The listing builds one solid part. Answer for the finished solid, in the listing's coordinates (mm). A direction names the side the tool comes from. Coordinates: 2 decimals unless noted, no trailing zeros. Write each loop counter-clockwise with the first axis right and the second up, starting at its lowest first coordinate (ties: lowest second). Pieces come first, ordered by that corner, then holes. Notation, with made-up numbers: M 18,79.5 L 53,79.5 A31 cw 53,105.5 Z; hole C 86,7 d2. An arc over 180 degrees is marked long. Answer as a JSON object with one key per item and string values. Group by question number.
from build123d import *

# Parameters (mm, degrees)
SKETCH2_R               = 101.6
BOSS_EXTRUDE1_DEPTH     = 76.2
SKETCH3_R               = 19.05
BOSS_EXTRUDE2_DEPTH     = 330.2
SKETCH12_R              = 20.32
BOSS_EXTRUDE5_DEPTH     = 7.62
BOSS_EXTRUDE6_OUTLINE_R = 19.05
BOSS_EXTRUDE6_DEPTH     = 35.56
SKETCH14_R              = 20.32
BOSS_EXTRUDE7_DEPTH     = 7.62
BOSS_EXTRUDE8_OUTLINE_R = 19.05
BOSS_EXTRUDE8_DEPTH     = 254
SKETCH16_R              = 101.6
BOSS_EXTRUDE9_DEPTH     = 76.2


# Read off the part's stored shape, not the designer's step: Boss-Extrude6, Boss-Extrude8
with BuildPart() as part:
    # Sketch2 → Boss-Extrude1 (new body)
    with BuildSketch(Plane.XY):
        with Locations(Location((0, 0, 0), (0, 0, 180))):
            Circle(SKETCH2_R)
    extrude(amount=BOSS_EXTRUDE1_DEPTH)

    # Sketch3 → Boss-Extrude2 (add)
    with BuildSketch(Plane.XY):
        Circle(SKETCH3_R)
    extrude(amount=BOSS_EXTRUDE2_DEPTH)

    # Sketch12 → Boss-Extrude5 (add)
    with BuildSketch(Plane.XY.offset(330.2)):
        with Locations(Location((0, 0, 0), (0, 0, 180))):
            Circle(SKETCH12_R)
    extrude(amount=BOSS_EXTRUDE5_DEPTH)

    # Boss-Extrude6 outline → Boss-Extrude6 (add)
    with BuildSketch(Plane.XY.offset(337.82)):
        Circle(BOSS_EXTRUDE6_OUTLINE_R)
    extrude(amount=BOSS_EXTRUDE6_DEPTH)

    # Sketch14 → Boss-Extrude7 (add)
    with BuildSketch(Plane.XY.offset(373.38)):
        with Locations(Location((0, 0, 0), (0, 0, 180))):
            Circle(SKETCH14_R)
    extrude(amount=BOSS_EXTRUDE7_DEPTH)

    # Boss-Extrude8 outline → Boss-Extrude8 (add)
    with BuildSketch(Plane.XY.offset(381)):
        Circle(BOSS_EXTRUDE8_OUTLINE_R)
    extrude(amount=BOSS_EXTRUDE8_DEPTH)

    # Sketch16 → Boss-Extrude9 (add)
    with BuildSketch(Plane.XY.offset(635)):
        with Locations(Location((0, 0, 0), (0, 0, 180))):
            Circle(SKETCH16_R)
    extrude(amount=BOSS_EXTRUDE9_DEPTH)


solid = part.part
Item 1: Consider L1, parallel to Z at x = 7, y = -47; L2, parallel to X at y = 1, z = 520; L3, parallel to Y at x = 2.5, z = 63. Determine where each line is inside the solid, lowest interval first. Write a range as from..to.
Item 2: A cutting plane is placed at B-B, the plane x = 0. Write down the section's boundary in (y, z), and give its area (3 significant figures).
Item 3: For a pull along Z with two mould halves and no side action, classify faces 3 (the face through (2.645, -20.147, 377.137)), 4 (the face through (-1, 1, 0)), 5 (the face through (-46.88, 90.14, 37.57)) as +Z half, -Z half, draft (parallel to the pull), parting line (faces both ways), or undercut.
Item 4: A cutting plane is placed at A-A, the plane y = -40. Write down the section's boundary in (x, z), and give its area (3 significant figures).
Item 5: A tool of negligible diameter and unlimited length cuts with its end or side. For faces 1 (the face through (-15.12, -11.59, 355.35)), 2 (the face through (-46.88, 90.14, 672.57)), from which of +Z, -Z, +X, -X, +Y, -Y can it reach the whole face along a straight path? Write none if from no direction.
Item 6: Flat-ended cylindrical pins translate along their axes: pin 1 Ø10 at (y, z) = (17.5, 550.5) entering from -X; pin 2 Ø12 at (y, z) = (18.5, 359.5) entering from +X. Find the tip coordinate at first contact, or state that the pin passes through.
Item 7: A cutting plane is placed at C-C, the plane x = -28. Write down the section's boundary in (y, z), and give its area (3 significant figures).
Answer:
{
 "1": {"L1": "0..76.2, 635..711.2", "L2": "-19.02..19.02", "L3": "-101.57..101.57"},
 "2": {"outline": "M -101.6,0 L 101.6,0 L 101.6,76.2 L 19.05,76.2 L 19.05,330.2 L 20.32,330.2 L 20.32,337.82 L 19.05,337.82 L 19.05,373.38 L 20.32,373.38 L 20.32,381 L 19.05,381 L 19.05,635 L 101.6,635 L 101.6,711.2 L -101.6,711.2 L -101.6,635 L -19.05,635 L -19.05,381 L -20.32,381 L -20.32,373.38 L -19.05,373.38 L -19.05,337.82 L -20.32,337.82 L -20.32,330.2 L -19.05,330.2 L -19.05,76.2 L -101.6,76.2 Z", "area": "52,300 mm2"},
 "3": {"face 3": "undercut", "face 4": "-Z half", "face 5": "draft"},
 "4": {"outline": "M -93.39,0 L 93.39,0 L 93.39,76.2 L -93.39,76.2 Z; M -93.39,635 L 93.39,635 L 93.39,711.2 L -93.39,711.2 Z", "area": "28,500 mm2"},
 "5": {"face 1": "none", "face 2": "+Z, -Z"},
 "6": {"pin 1": "x = -14.38", "pin 2": "x = 14.38"},
 "7": {"outline": "M -97.67,0 L 97.67,0 L 97.67,76.2 L -97.67,76.2 Z; M -97.67,635 L 97.67,635 L 97.67,711.2 L -97.67,711.2 Z", "area": "29,800 mm2"}
}
